Geometry: final body of the model. Coordinates: model frame, mm. Face numbers are marked on the shaded views. A direction names the side the tool comes from. Give positions to 0.01 mm unless a question says otherwise; leave off trailing zeros. Write each loop counter-clockwise with the first axis right and the second up, starting at its lowest first coordinate (ties: lowest second). Pieces come first, ordered by that corner, then holes. Notation, with made-up numbers: M 53.5,65.5 L 87.5,65.5 A5 ccw 87.5,71.5 Z; hole C 8.5,81.25 d10. An arc over 180 degrees is marked long. Use a Markdown table: item, result. Add a question column.
1) Section B-B on y = 1.5. Return the cut outline in (x, z) (3 decimals).
2) Section C-C on x = 0. Return the cut outline in (y, z).
3) Section A-A on x = -21. Return the cut outline in (y, z), then the cut area to 3 significant figures.
4) Draft query along Z for the marked faces 1, 2, 3 and 4. Return one class per face: +Z half, -Z half, draft (parallel to the pull), parting line (faces both ways), or undercut.
5) Section D-D on y = -30.5. Return the cut outline in (x, z), then the cut area to 3 significant figures.
6) Set-up query: the marked faces 5, 6 and 7. Return all of +Z, -Z, +X, -X, +Y, -Y with unobstructed straight access to the full face (end or side cutting, diameter ignored); none if empty.
7) Line query: line 1 (X direction, y = -13, z = 15.25); line 2 (Z direction, x = 25.5, y = 26); line 3 (Y direction, x = -17, z = 20.75). Output: solid intervals per line, ascending.
8) Pin query (flat end, axial travel): pin 1 (5 mm diameter, centred on x = -21.5, z = 14, fed in from -Y); pin 2 (3.5 mm diameter, centred on x = -16.5, z = 11.5, fed in from +Y); pin 3 (4 mm diameter, centred on x = -8, z = 22.5, fed in from +Y). Return the tip coordinate at first contact, or that it passes through.
```python
from build123d import *

# Parameters (mm, degrees)
F0_R      = 30
F0_R_2    = 25.169146
F1_DEPTH  = 26
F0_R_3    = 45
F2_DEPTH  = 3
F3_R      = 45
F3_R_2    = 30
F4_DEPTH  = 3
F5_R      = 47.552923
F5_R_2    = 45
F6_DEPTH  = 26
F8_DEPTH  = 26
F9_W      = 10.5
F9_H      = 26
F9_W_2    = 3
F10_DEPTH = 36
F11_W     = 10.5
F11_H     = 26
F12_DEPTH = 25


with BuildPart() as f1:
    # F0 (on Top) → F1 (new body)
    with BuildSketch(Plane.XY):
        Circle(F0_R)
        Circle(F0_R_2, mode=Mode.SUBTRACT)
    extrude(amount=F1_DEPTH)

    # F0 (on Top) → F2 (join)
    with BuildSketch(Plane.XY):
        Circle(F0_R_3)
        Circle(F0_R, mode=Mode.SUBTRACT)
    extrude(amount=F2_DEPTH)

    # F3 (on face) → F4 (join)
    with BuildSketch(Plane.XY.offset(26)):
        Circle(F3_R)
        Circle(F3_R_2, mode=Mode.SUBTRACT)
    extrude(amount=-F4_DEPTH)

    # F5 (on face) → F6 (join)
    with BuildSketch(Plane(origin=(0, 0, 0), x_dir=(1, 0, 0), z_dir=(0, 0, -1))):
        Circle(F5_R)
        Circle(F5_R_2, mode=Mode.SUBTRACT)
    extrude(amount=-F6_DEPTH)

    # F7 (on face) → F8 (cut)
    with BuildSketch(Plane(origin=(0, 0, 0), x_dir=(1, 0, 0), z_dir=(0, 0, -1))):
        with BuildLine():
            Line((25.169146, 0), (47.552923, 0))
            ThreePointArc((47.552923, 0), (0, 47.552923), (-47.552923, 0))
            Line((-47.552923, 0), (-25.169146, 0))
            ThreePointArc((-25.169146, 0), (0, 25.169146), (25.169146, 0))
        make_face()
    extrude(amount=-F8_DEPTH, mode=Mode.SUBTRACT)

    # F9 (on face) → F10 (join)
    with BuildSketch(Plane.XZ):
        with Locations((-21.75, 13)):
            Rectangle(F9_W, F9_H)
        with Locations((-15, 13)):
            Rectangle(F9_W_2, F9_H)
        with Locations((-28.5, 13)):
            Rectangle(F9_W_2, F9_H)
    extrude(amount=F10_DEPTH)

    # F11 (on face) → F12 (cut)
    with BuildSketch(Plane.XZ.offset(36)):
        with Locations((-21.75, 13)):
            Rectangle(F11_W, F11_H)
    extrude(amount=-F12_DEPTH, mode=Mode.SUBTRACT)


solid = f1.part
```
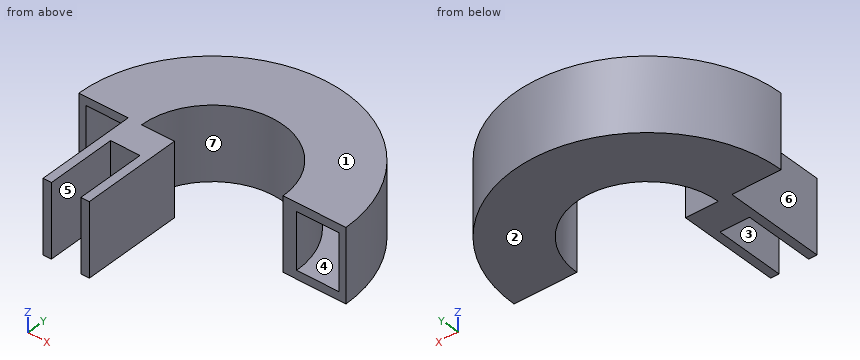
Found:
| question | item | result |
|---|---|---|
| 1 | outline | M -47.529,0 L -25.124,0 L -25.124,26 L -47.529,26 Z; M 25.124,0 L 47.529,0 L 47.529,26 L 25.124,26 Z; hole M -44.975,3 L -29.962,3 L -29.962,23 L -44.975,23 Z; hole M 29.962,3 L 44.975,3 L 44.975,23 L 29.962,23 Z |
| 2 | outline | M 25.17,0 L 47.55,0 L 47.55,26 L 25.17,26 Z; hole M 30,3 L 45,3 L 45,23 L 30,23 Z |
| 3 | outline | M -11,0 L 0,0 L 0,26 L -11,26 Z; M 13.87,0 L 42.66,0 L 42.66,26 L 13.87,26 Z; hole M 21.42,3 L 39.8,3 L 39.8,23 L 21.42,23 Z |
| 3 | area | 667 mm² |
| 4 | face 1 | +Z half |
| 4 | face 2 | -Z half |
| 4 | face 3 | draft |
| 4 | face 4 | undercut |
| 5 | outline | M -30,0 L -27,0 L -27,26 L -30,26 Z; M -16.5,0 L -13.5,0 L -13.5,26 L -16.5,26 Z |
| 5 | area | 156 mm² |
| 6 | face 5 | +Z, -Z, -Y |
| 6 | face 6 | +Z, -Z, -X, -Y |
| 6 | face 7 | +Z, -Z |
| 7 | line 1 | -30 to -27, -16.5 to -13.5 |
| 7 | line 2 | 0 to 3, 23 to 26 |
| 7 | line 3 | -11 to 0, 18.56 to 24.72, 41.67 to 44.41 |
| 8 | pin 1 | y = -11 |
| 8 | pin 2 | y = 45.21 |
| 8 | pin 3 | y = 47.17 |
